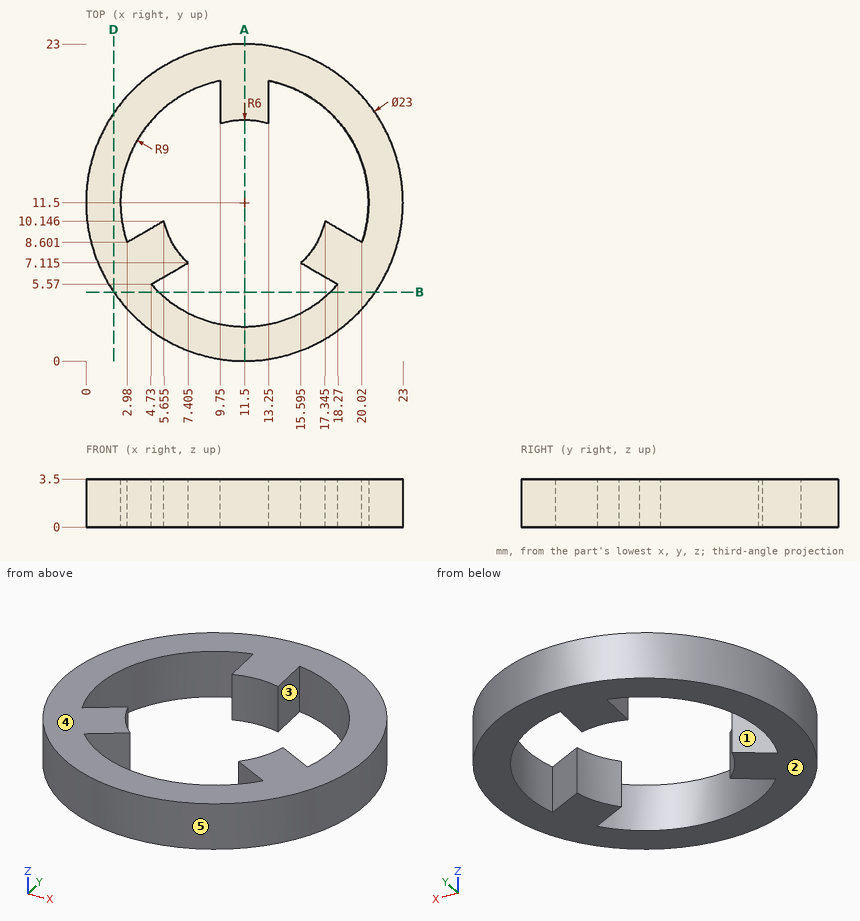
The figure shows three views and two pictorial views of one solid part (mm, origin at its lowest corner). Answer the questions. A direction names the side the tool comes from. Round coordinates to 2 decimals unless told otherwise and drop trailing zeros. Write each loop counter-clockwise with the first axis right and the second up, starting at its lowest first coordinate (ties: lowest second). Pieces come first, ordered by that corner, then holes. Notation, with made-up numbers: M -11,86.5 L 1,86.5 A12 ccw 1,102.5 Z; hole C 2,69 d8. An arc over 180 degrees is marked long. Write each question's results on one line, items separated by ' | '. Start each with the question number.
(1) Find the intervals of material crossed by line 1 (X direction, y = 9.75, z = 2.85) (1 decimal); line 2 (Y direction, x = 7, z = 0.9) (1 decimal); line 3 (Y direction, x = 6.5, z = 2.8) (1 decimal), in increasing order.
(2) Determine the mould class of the marked faces 3, 4 and 5 for opening direction X: +X half, -X half, draft (parallel to the pull), parting line (faces both ways), or undercut.
(3) For the marked faces 1 and 2, determine the directions among +Z, -Z, +X, -X, +Y, -Y from which every point of the face is accessible in a straight line to the end or side of a thin tool.
(4) The part is cut by section B-B, the plane y = 5. Write down the section's boundary in (x, z) (1 decimal).
(5) Each of these flat-tipped pins is pushed along its axis until it touches: P1, Ø1.5, axis at x = 18, z = 0.5, coming from the +Y side; P2, Ø1, axis at x = 2.5, z = 1, coming from the -Y side (1 decimal); P3, Ø0.9, axis at y = 19.5, z = 1.5, coming from the +X side (1 decimal). Where does it stop, or does it pass through?
(6) The part is cut by section D-D, the plane x = 2. Write down the section's boundary in (y, z).
(7) The part is cut by section A-A, the plane x = 11.5. Write down the section's boundary in (y, z), and give its area (3 significant figures).
Worked answers:
1) line 1: x = 0.1 to 2.7, 5 to 5.8, 17.2 to 18, 20.3 to 22.9 | line 2: y = 0.9 to 3.7, 6.9 to 7.5, 19.3 to 22.1 | line 3: y = 1.1 to 4, 6.6 to 8.2, 19 to 21.9
2) face 3: undercut | face 4: draft | face 5: parting line
3) face 1: +Z, -Z | face 2: -Z, +X, -X, +Y, -Y
4) outline: M 2,0 L 5.3,0 L 5.3,3.5 L 2,3.5 Z; M 17.7,0 L 21,0 L 21,3.5 L 17.7,3.5 Z
5) P1: stops at y = 21.46 | P2: stops at y = 3.8 | P3: stops at x = 20.2
6) outline: M 5.02,0 L 17.98,0 L 17.98,3.5 L 5.02,3.5 Z
7) outline: M 0,0 L 2.5,0 L 2.5,3.5 L 0,3.5 Z; M 17.5,0 L 23,0 L 23,3.5 L 17.5,3.5 Z | area: 28.0 mm²
